Design review of the part shown in the three views and the two pictorial views. Dimensions are in mm from the part's minimum x, y and z. Round coordinates to 2 decimals unless told otherwise and drop trailing zeros. Order: outer loops, then holes, each group sorted by start corner. A loop starts at its lowest first (then second) coordinate and runs counter-clockwise, first axis right, second up. Notation, with made-up numbers: (72.5, -9.5) - (82.5, -9.5) arc R20 ccw to (82.5, 18.5) - close; hole circle Ø7 at (-34, 36). An arc over 180 degrees is marked (long way). Use CSV: the item, a comma, the result in double quotes.
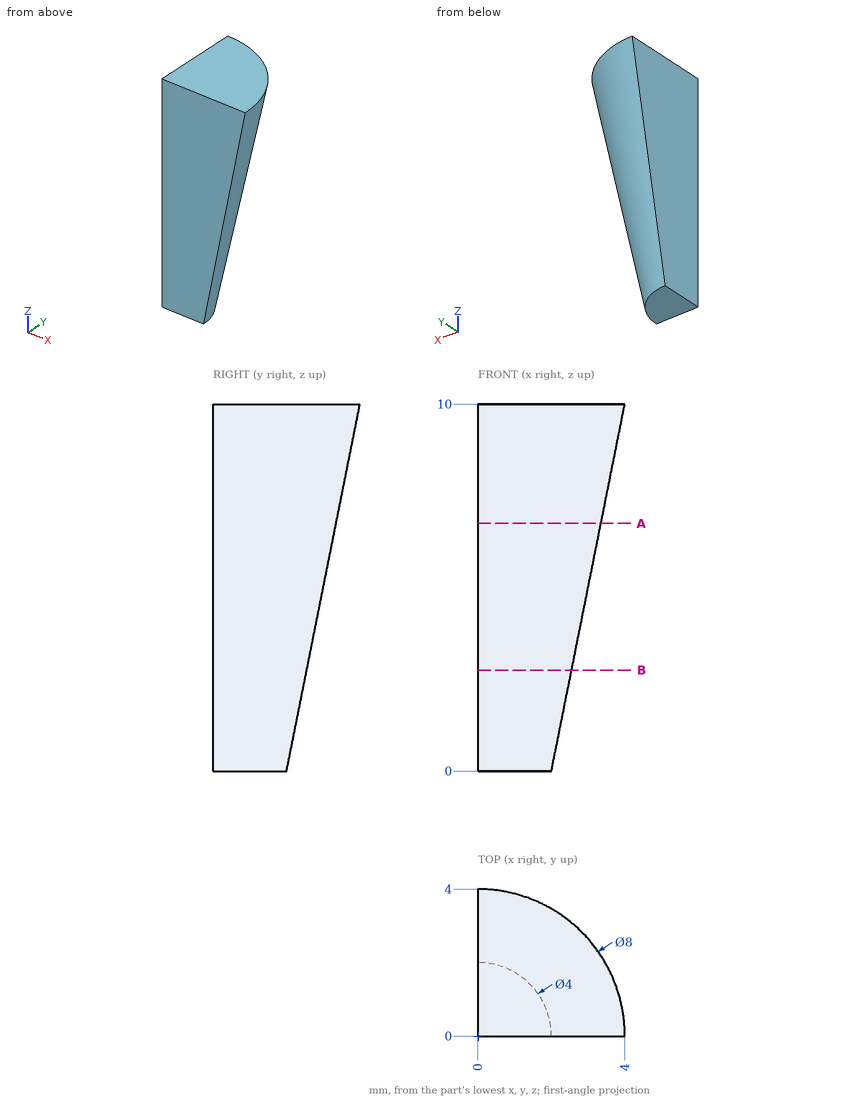
1) Insertion check: pin 1 Ø1.5 at (x, z) = (1, 3) entering from +Y. The pin has a flat end and moves straight along its axis. Give the tip position at first contact, or say it passes through.
Data:
pin 1,"stops at y = 2.67"
2) We need section A-A (z = 6.75). Give the boundary of the cut face in (x, y).
Data:
outline,"(0, 0) - (3.35, 0) arc R3.35 ccw to (0, 3.35) - close"
3) We need section B-B (z = 2.75). Give the boundary of the cut face in (x, y), then the cut area to 3 significant figures.
Data:
outline,"(0, 0) - (2.55, 0) arc R2.55 ccw to (0, 2.55) - close"
area,"5.11 mm2"
4) To check wall thickness, follow L1, parallel to Y at x = 0.9, z = 7; L2, parallel to Y at x = 1.1, z = 3.75; L3, parallel to X at y = 1.65, z = 9. State the ranges of each line that lie inside material, in increasing order. Write a range as from..to.
Data:
L1,"y = 0..3.28"
L2,"y = 0..2.52"
L3,"x = 0..3.42"
